Here's how the part is built. I have some questions about the finished solid (model axes, mm). A direction names the side the tool comes from. Round coordinates to 2 decimals unless told otherwise and drop trailing zeros. Write each loop counter-clockwise with the first axis right and the second up, starting at its lowest first coordinate (ties: lowest second). Pieces come first, ordered by that corner, then holes. Notation, with made-up numbers: (-6, 59.25) -> (49, 59.25) arc R34 cw to (49, 91.25) -> close; hole circle Ø4 at (8, 72.5). An arc over 180 degrees is marked (long way). Answer as CSV lines item,"result".
Autodesk Inventor part; units mm, degrees
ref_plane "YZ Plane" through (0, 0, 0) normal (1, 0, 0) x (0, 1, 0)
ref_plane "XZ Plane" through (0, 0, 0) normal (0, 1, 0) x (-1, 0, 0)
ref_plane "XY Plane" through (0, 0, 0) normal (0, 0, 1) x (1, 0, 0)
sketch "Sketch1" plane through (0, 0, 0) normal (0, 1, 0) x (-1, 0, 0)
  circle A0 centre (0, 0) radius 4.5
  dimension "d0" = 9
extrude "Extrusion1" add sketch "Sketch1" along normal blind 10
fillet "Fillet1" radius 4.5 1 edges at (4.5, 10, 0)
sketch "Sketch2" plane through (0, 0, 0) normal (0, -1, 0) x (1, 0, 0)
  line L0 (0, 2.5) -> (30, 2.5)
  line L1 (30, 2.5) -> (30, -2.5)
  line L2 (30, -2.5) -> (0, -2.5)
  line L3 (0, -2.5) -> (0, 2.5)
  point P0 (0, 0)
  dimension "d4" = 30
  dimension "d5" = 5
  dimension "d6" = 2.5
extrude "Extrusion2" add sketch "Sketch2" against normal blind 0.2
sketch "Sketch3" plane through (0, 0, 0) normal (0, -1, 0) x (1, 0, 0)
  line L0 (30, 2.5) -> (3.7417, 2.5)
  circle A0 centre (35.5, 0) radius 10
  circle A1 centre (0, 0) radius 0.101
  circle A2 centre (35.5, 0) radius 5
  line L1 (30, 2.5) -> (30, -2.5)
  point P0 (4.3301, 2.5)
  dimension "d20" = 10
  dimension "d21" = 5
  dimension "d22" = 5.5
extrude "Extrusion3" add sketch "Sketch3" against normal blind 5 contours A0
fillet "Fillet2" radius 2 4 edges at (25.5, 5, 0) (25.5, 0.2, 0) (25.8175, 0.1, -2.5) (25.8175, 0.1, 2.5)
properties part number "pipe form"
1. Suppose I cut it at B-B on z = 0. Please give me the cut outline in (x, y), and give its area (3 significant figures).
Numbers:
outline,"(-4.5, 0) -> (30.5, 0) -> (30.5, 5) -> (27.5, 5) arc R2 ccw to (25.5, 3) -> (25.5, 2.2) arc R2 cw to (23.5, 0.2) -> (4.5, 0.2) -> (4.5, 5.5) arc R4.5 ccw to (-4.5, 5.5) -> close; (40.5, 0) -> (45.5, 0) -> (45.5, 3) arc R2 ccw to (43.5, 5) -> (40.5, 5) -> close"
area,"135 mm^2"
2. Suppose I cut it at A-A on x = 35.5. Please give me the cut outline in (y, z), and give its area (3 significant figures).
Numbers:
outline,"(0, -10) -> (3, -10) arc R2 ccw to (5, -8) -> (5, -5) -> (0, -5) -> close; (0, 5) -> (5, 5) -> (5, 8) arc R2 ccw to (3, 10) -> (0, 10) -> close"
area,"48.3 mm^2"
3. On a 3-axis mill with a long thin cutter (end or side, diameter ignored), from which of +Z, -Z, +X, -X, +Y, -Y can I reach the whole of each face in a straight line? I mean faces 3 (the face through (30.505, 2.465, 0.22)), 4 (the face through (25.7, 0.6, -3)), 5 (the face through (25.7, 0.6, 3)). Say none if no direction works.
Numbers:
face 3,"+Y, -Y"
face 4,"-Z, +Y, -Y"
face 5,"+Z, +Y, -Y"
4. For pin 1 Ø2.5 at (x, z) = (12.5, -0.5) entering from +Y; pin 2 Ø1 at (x, z) = (2, 2) entering from -Y; pin 3 Ø8 at (x, z) = (37, -2.5) entering from +Y, each with a flat end and sliding along its axis, tell me the tip position at first contact or that it passes through.
Numbers:
pin 1,"stops at y = 0.2"
pin 2,"stops at y = 0"
pin 3,"stops at y = 5"
5. Suppose I cut it at C-C on y = 4.25. Please give me the cut outline in (x, z), and give its area (3 significant figures).
Numbers:
outline,"circle Ø9 at (0, 0); circle Ø19.12 at (35.5, 0); hole circle Ø10 at (35.5, 0)"
area,"272 mm^2"
6. Suppose I cut it at D-D on x = 0. Please give me the cut outline in (y, z), and give its area (3 significant figures).
Numbers:
outline,"(0, -4.5) -> (5.5, -4.5) arc R4.5 ccw to (5.5, 4.5) -> (0, 4.5) -> close"
area,"81.3 mm^2"
7. If I drill on line 1 (X direction, y = 2.25, z = -3.5); line 2 (X direction, y = 4.25, z = -2.5); line 3 (Z direction, x = 35.5, y = 2.45), over which ranges is the centre line in solid material (lowest first)?
Numbers:
line 1,"x = -2.83 to 2.83, 26.13 to 31.93, 39.07 to 44.87"
line 2,"x = -3.74 to 3.74, 26.27 to 31.17, 39.83 to 44.73"
line 3,"z = -10 to -5, 5 to 10"
8. If we mould it in two halves opening along X, with no side actions, what happens to faces 1 (the face through (39, 5, 4)), 2 (the face through (0.59, 2.71, -4.46))? For each: released by +X, released by -X, zero draft, split by the parting line, or undercut.
Numbers:
face 1,"zero draft"
face 2,"undercut"
